from build123d import *

# Parameters (mm, degrees)
EXTRUDE_1_DEPTH = 3


with BuildPart() as part:
    # 草图2 → 凸台-拉伸1 (new body)
    with BuildSketch(Plane(origin=(0, 0, 0), x_dir=(1, 0, 0), z_dir=(0, 1, 0))):
        with BuildLine():
            Line((-25, 27.5), (-20, 27.5))
            Line((-20, 27.5), (-20, 30.5))
            Line((-20, 30.5), (-10, 30.5))
            Line((-10, 30.5), (-10, 27.5))
            Line((-10, 27.5), (-5, 27.5))
            Line((-5, 27.5), (-5, 30.5))
            Line((-5, 30.5), (5, 30.5))
            Line((5, 30.5), (5, 27.5))
            Line((5, 27.5), (10, 27.5))
            Line((10, 27.5), (10, 30.5))
            Line((10, 30.5), (20, 30.5))
            Line((20, 30.5), (20, 27.5))
            Line((20, 27.5), (25, 27.5))
            Line((25, 27.5), (25, 20))
            Line((25, 20), (28, 20))
            Line((28, 20), (28, 10))
            Line((28, 10), (25, 10))
            Line((25, 10), (25, 5))
            Line((25, 5), (28, 5))
            Line((28, 5), (28, 0.5))
            Line((28, 0.5), (28, 0))
            Line((28, 0), (21, 0))
            Line((21, 0), (21, 0.5))
            ThreePointArc((21, 0.5), (0, 21.5), (-21, 0.5))
            Line((-21, 0.5), (-21, 0))
            Line((-21, 0), (-28, 0))
            Line((-28, 0), (-28, 0.5))
            Line((-28, 0.5), (-28, 5))
            Line((-28, 5), (-25, 5))
            Line((-25, 5), (-25, 10))
            Line((-25, 10), (-28, 10))
            Line((-28, 10), (-28, 20))
            Line((-28, 20), (-25, 20))
            Line((-25, 20), (-25, 27.5))
        make_face()
    extrude(amount=EXTRUDE_1_DEPTH)


solid = part.part
The model under review builds one solid part; all positions refer to its coordinate system, in mm. A direction names the side the tool comes from. Round coordinates to 2 decimals unless told otherwise and drop trailing zeros. Loops run counter-clockwise (first coordinate to the right, second up) from the corner with the lowest first, then second, coordinate; pieces in that order, holes last. Notation, with made-up numbers: (51, 61) -> (55, 61) arc R25 cw to (55, 79) -> close; hole circle Ø4 at (20.5, 18). An arc over 180 degrees is marked (long way). Return JSON: item names as keys, results as strings.
(1) Add section A-A on z = -3. Write out the cut boundary in (x, y).
Solved:
{"outline": "(-28, 0) -> (-20.85, 0) -> (-20.85, 3) -> (-28, 3) -> close; (20.85, 0) -> (28, 0) -> (28, 3) -> (20.85, 3) -> close"}
(2) For faces 1 (the flat face through (25, 1, -24)), 2 (the flat face through (26, 1, -5)), 3 (the flat face through (-25, 1, -24)), 4 (the flat face through (-27, 1, -5)), list the 3-axis set-ups (+Z, -Z, +X, -X, +Y, -Y) from which the entire face can be reached by the end or side of a thin tool; tool diameter is ignored.
Solved:
{"face 1": "-Z, +X, +Y, -Y", "face 2": "+X, +Y, -Y", "face 3": "-Z, -X, +Y, -Y", "face 4": "-X, +Y, -Y"}
(3) For line 1 (X direction, y = 1.1, z = -28.5); line 2 (Z direction, x = 22, y = 0.6); line 3 (X direction, y = 1.2, z = -4.5), list the stretches that pass through material, from the lowest coordinate up.
Solved:
{"line 1": "-20 to -10, -5 to 5, 10 to 20", "line 2": "-27.5 to 0", "line 3": "-28 to -20.62, 20.62 to 28"}
(4) Add section C-C on x = 0. Write out the cut boundary in (y, z), plus the area to 3 significant figures.
Solved:
{"outline": "(0, -30.5) -> (3, -30.5) -> (3, -21.5) -> (0, -21.5) -> close", "area": "27.0 mm2"}
(5) For pin 1 (0.9 mm diameter, centred on y = 2, z = -29.5, fed in from -X); pin 2 (1.5 mm diameter, centred on x = 6.5, y = 1, fed in from -Z); pin 3 (12 mm diameter, centred on x = -1.5, z = -25, fed in from -Y); pin 4 (1.5 mm diameter, centred on y = 2, z = -29, fed in from +X), all flat-tipped, find the tip position at first contact; note any pin that passes through.
Solved:
{"pin 1": "x = -20", "pin 2": "z = -27.5", "pin 3": "y = 0", "pin 4": "x = 20"}
(6) Add section D-D on z = -17.5. Write out the cut boundary in (x, y), plus the area to 3 significant figures.
Solved:
{"outline": "(-28, 0) -> (-12.33, 0) -> (-12.33, 3) -> (-28, 3) -> close; (12.33, 0) -> (28, 0) -> (28, 3) -> (12.33, 3) -> close", "area": "94.0 mm2"}
(7) The part is to be moulded in two halves that separate along Z. For faces 5 (the flat face through (-24, 1, 0)), 6 (the flat face through (-25, 1, -7)), 7 (the flat face through (5, 1, -29)), say which applies: released by +Z, released by -Z, zero draft, split by the parting line, or undercut.
Solved:
{"face 5": "released by +Z", "face 6": "undercut", "face 7": "zero draft"}
